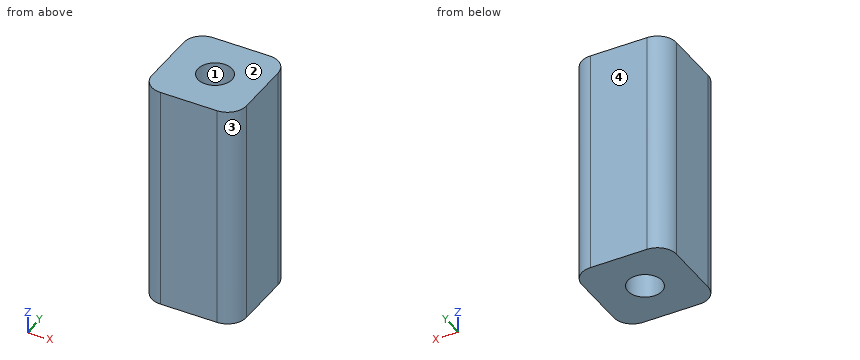
```python
from build123d import *

# Parameters (mm, degrees)
SKETCH1_W            = 10
SKETCH1_H            = 10
BOSS_EXTRUDE1_DEPTH  = 24
M3_CLEARANCE_HOLE1_D = 3.6
FILLET1_R            = 2


with BuildPart() as part:
    # Sketch1 → Boss-Extrude1 (new body)
    with BuildSketch(Plane.XY):
        Rectangle(SKETCH1_W, SKETCH1_H)
    extrude(amount=BOSS_EXTRUDE1_DEPTH)

    # M3 Clearance Hole1 (through all)
    with Locations(Plane.XY.offset(24)):
        with Locations((0, 0)):
            Hole(M3_CLEARANCE_HOLE1_D / 2)

    # Fillet1
    fillet1_edges = [part.edges().sort_by_distance(p)[0] for p in [
        (5, -5, 12),
        (-5, -5, 12),
        (-5, 5, 12),
        (5, 5, 12),
    ]]
    fillet(fillet1_edges, radius=FILLET1_R)


solid = part.part
```
For this review, take the finished solid that the model builds, in its own axes (mm). Face numbers are marked on the shaded views. Round coordinates to 2 decimals unless told otherwise and drop trailing zeros. Order: outer loops, then holes, each group sorted by start corner. A loop starts at its lowest first (then second) coordinate and runs counter-clockwise, first axis right, second up. Notation, with made-up numbers: (2, 71) -> (7, 71) arc R17 cw to (7, 85) -> close; hole circle Ø4 at (46.5, -32.5). An arc over 180 degrees is marked (long way). Use a Markdown table: item, result.
Item 1: Draft analysis for pull direction Y (two halves, no side actions). For the marked faces 1, 2, 3 and 4, state which applies: +Y half, -Y half, draft (parallel to the pull), parting line (faces both ways), or undercut.
Resolved:
| item | result |
|---|---|
| face 1 | undercut |
| face 2 | draft |
| face 3 | -Y half |
| face 4 | +Y half |
Item 2: Take a section at A-A (y = 0). State the section outline as (x, z) points, plus the area to 3 significant figures.
Resolved:
| item | result |
|---|---|
| outline | (-5, 0) -> (-1.8, 0) -> (-1.8, 24) -> (-5, 24) -> close; (1.8, 0) -> (5, 0) -> (5, 24) -> (1.8, 24) -> close |
| area | 154 mm² |
Item 3: Take a section at C-C (z = 5). State the section outline as (x, y) points.
Resolved:
| item | result |
|---|---|
| outline | (-5, -3) arc R2 ccw to (-3, -5) -> (3, -5) arc R2 ccw to (5, -3) -> (5, 3) arc R2 ccw to (3, 5) -> (-3, 5) arc R2 ccw to (-5, 3) -> close; hole circle Ø3.6 at (0, 0) |
Item 4: For line 1 along Y through (x, z) = (0, 6); line 2 along X through (y, z) = (-1, 13); line 3 along Y through (x, z) = (0.75, 16.5), list the stretches that pass through material, from the lowest coordinate up. Write a range as [from, to].
Resolved:
| item | result |
|---|---|
| line 1 | y = [-5, -1.8], [1.8, 5] |
| line 2 | x = [-5, -1.5], [1.5, 5] |
| line 3 | y = [-5, -1.64], [1.64, 5] |
Item 5: For pin 1 (6 mm diameter, centred on x = 1, y = 3, fed in from -Z), flat-tipped, find the tip position at first contact; note if it passes through.
Resolved:
| item | result |
|---|---|
| pin 1 | stops at z = 0 |
Item 6: Take a section at D-D (x = 4). State the section outline as (y, z) points, plus the area to 3 significant figures.
Resolved:
| item | result |
|---|---|
| outline | (-4.73, 0) -> (4.73, 0) -> (4.73, 24) -> (-4.73, 24) -> close |
| area | 227 mm² |
